from build123d import *

# Parameters (mm, degrees)
F0_R     = 1.27
F1_DEPTH = 7.62
F2_R     = 2.54
F3_DEPTH = 2.54
F4_W     = 1.27
F4_H     = 3.81
F5_DEPTH = 1.27


# Not quite as in the source:
# - a fillet or chamfer that OpenCascade refuses, or shapes differently, is made with other operations: its cross-section is extruded or revolved along the edge and cut away or added


with BuildPart() as f1:
    # F0 (on Top) → F1 (new body)
    with BuildSketch(Plane.XY):
        Circle(F0_R)
    extrude(amount=F1_DEPTH)

    # F2 (on face) → F3 (join)
    with BuildSketch(Plane.XY.offset(7.62)):
        Circle(F2_R)
    extrude(amount=F3_DEPTH)

    # F4 (on face) → F5 (cut)
    with BuildSketch(Plane.XY.offset(10.16)):
        Rectangle(F4_W, F4_H)
    extrude(amount=-F5_DEPTH, mode=Mode.SUBTRACT)

    # F6: fillet of radius 1.905 on 1 edges, made by hand

    # F6_s1 → F6_t2 (revolve, cut)
    with BuildSketch(Plane.XZ):
        with BuildLine():
            ThreePointArc((2.54, 8.255), (1.9820384182, 9.6020384182), (0.635, 10.16))
            Line((0.635, 10.16), (2.54, 10.16))
            Line((2.54, 10.16), (2.54, 8.255))
        make_face()
    revolve(axis=Axis((0, 0, 10.16), (0, 0, 1)), mode=Mode.SUBTRACT)


solid = f1.part
Can you work these out from the model? Positions are in its coordinate system, mm. A direction names the side the tool comes from. Coordinates: 2 decimals unless noted, no trailing zeros. Write each loop counter-clockwise with the first axis right and the second up, starting at its lowest first coordinate (ties: lowest second). Pieces come first, ordered by that corner, then holes.
Q1. Which directions (+Z, -Z, +X, -X, +Y, -Y) give clear straight access to the entire face, cutting with the end or side of a thin tool? Please do faces 5 (the face through (0.635, 0, 10)), 6 (the face through (-0.33, 2.52, 7.93)).
Results found:
face 5: +Z
face 6: +Z, -Z
Q2. Imagine slicing it at B-B, the plane z = 8. List the corners of the cut face in (x, y) for me, plus the area to 3 significant figures.
Results found:
outline: circle Ø5.08 at (0, 0)
area: 20.3 mm2
Q3. Please list where these lines run through material, in increasing order: L1, parallel to Y at x = -0.45, z = 9 (1 decimal); L2, parallel to Z at x = -0.55, y = 0.45; L3, parallel to Z at x = 1.3, y = 1.5.
Results found:
L1: y = -2.3 to -1.9, 1.9 to 2.3
L2: z = 0 to 8.89
L3: z = 7.62 to 9.6
Q4. For P1, Ø3, axis at y = -1.5, z = 9, coming from the -X side; P2, Ø2, axis at x = -0.5, z = 1, coming from the -Y side; P3, Ø1, axis at x = -0.5, y = -1, coming from the +Z side; P4, Ø1, axis at y = 2, z = 3.5, coming from the -X side, each with a flat end and sliding along its axis, tell me the tip position at first contact or that it passes through.
Results found:
P1: stops at x = -2.53
P2: stops at y = -1.27
P3: stops at z = 10.15
P4: passes through
Q5. If we mould it in two halves opening along X, with no side actions, what happens to faces 1 (the face through (0, 0, 8.89)), 2 (the face through (1.1, -1.1, 7.62)), 3 (the face through (-0.17, 1.26, 3.76)), 4 (the face through (-0.635, 0, 10))? For each: +X half, -X half, draft (parallel to the pull), parting line (faces both ways), or undercut.
Results found:
face 1: undercut
face 2: draft
face 3: parting line
face 4: undercut
Q6. Imagine slicing it at A-A, the plane z = 4.75. List the corners of the cut face in (x, y) for me.
Results found:
outline: circle Ø2.54 at (0, 0)
